Geometry: final body of the model. Coordinates: model frame, mm. A direction names the side the tool comes from. Give positions to 0.01 mm unless a question says otherwise; leave off trailing zeros. Loops run counter-clockwise (first coordinate to the right, second up) from the corner with the lowest first, then second, coordinate; pieces in that order, holes last. Notation, with made-up numbers: (68, 31) -> (106, 31) arc R9 cw to (106, 36) -> close; hole circle Ø9 at (22.25, 78.5). An arc over 180 degrees is marked (long way). Answer in a Markdown table with one row per item. Add a question column.
1) First-contact query: P1, Ø0.8, axis at x = -12, z = 3.5, coming from the -Y side; P2, Ø2, axis at x = -22, y = -20, coming from the +Z side; P3, Ø9.5, axis at x = -12.5, y = -1, coming from the +Z side; P4, Ø0.8, axis at x = -1, z = 3.5, coming from the +Y side. Flat tips, straight axial feed; report the tip coordinate or a pass-through.
2) Draft query along Y for faces 4 (the flat face through (0, 30, 3)), 5 (the flat face through (0, -10, 3)), 6 (the flat face through (0, -35, 1)). Return one class per face: +Y half, -Y half, draft (parallel to the pull), parting line (faces both ways), or undercut.
3) Access query for faces 1 (the flat face through (0, 20, 3)), 2 (the flat face through (0, -30, 3)), 3 (the flat face through (-29.5, 0, 2)). Directions: +Z, -Z, +X, -X, +Y, -Y. A direction counts if a zero-diameter tool reaches every point of the face in a straight line with its end or side. Return the directions, or none.
4) Line query: line 1 (Z direction, x = -16, y = 17). Output: solid intervals per line, ascending. Write a range as from..to.
5) Section query A-A (y = 23). Return the cut outline in (x, z), plus the area to 3 significant figures.
```python
from build123d import *

# Parameters (mm, degrees)
SKETCH_W     = 59
SKETCH_H     = 70
PAD_DEPTH    = 3
SKETCH001_W  = 59
SKETCH001_H  = 0.5
PAD001_DEPTH = 1


with BuildPart() as part:
    # Sketch → Pad (new body)
    with BuildSketch(Plane.XY):
        Rectangle(SKETCH_W, SKETCH_H)
    extrude(amount=PAD_DEPTH)

    # Sketch001 (on Face6 of Pad) → Pad001 (join)
    with BuildSketch(Plane.XY.offset(3)):
        with Locations((0, -25.5)):
            Rectangle(SKETCH001_W, SKETCH001_H)
        with Locations((0, -24.5)):
            Rectangle(SKETCH001_W, SKETCH001_H)
        with Locations((0, -15.5)):
            Rectangle(SKETCH001_W, SKETCH001_H)
        with Locations((0, -14.5)):
            Rectangle(SKETCH001_W, SKETCH001_H)
        with Locations((0, -5.5)):
            Rectangle(SKETCH001_W, SKETCH001_H)
        with Locations((0, -4.5)):
            Rectangle(SKETCH001_W, SKETCH001_H)
        with Locations((0, 4.5)):
            Rectangle(SKETCH001_W, SKETCH001_H)
        with Locations((0, 5.5)):
            Rectangle(SKETCH001_W, SKETCH001_H)
        with Locations((0, 14.5)):
            Rectangle(SKETCH001_W, SKETCH001_H)
        with Locations((0, 15.5)):
            Rectangle(SKETCH001_W, SKETCH001_H)
        with Locations((0, 24.5)):
            Rectangle(SKETCH001_W, SKETCH001_H)
        with Locations((0, 25.5)):
            Rectangle(SKETCH001_W, SKETCH001_H)
    extrude(amount=PAD001_DEPTH)


solid = part.part
```
Evaluation:
| question | item | result |
|---|---|---|
| 1 | P1 | y = -25.75 |
| 1 | P2 | z = 3 |
| 1 | P3 | z = 4 |
| 1 | P4 | y = 25.75 |
| 2 | face 4 | draft |
| 2 | face 5 | undercut |
| 2 | face 6 | -Y half |
| 3 | face 1 | +Z, +X, -X |
| 3 | face 2 | +Z, +X, -X, -Y |
| 3 | face 3 | +Z, -Z, -X, +Y, -Y |
| 4 | line 1 | 0..3 |
| 5 | outline | (-29.5, 0) -> (29.5, 0) -> (29.5, 3) -> (-29.5, 3) -> close |
| 5 | area | 177 mm² |
